Build history of the part. All positions in model axes, mm. A direction names the side the tool comes from. Round coordinates to 2 decimals unless told otherwise and drop trailing zeros. Loops run counter-clockwise (first coordinate to the right, second up) from the corner with the lowest first, then second, coordinate; pieces in that order, holes last. Notation, with made-up numbers: M 10,2 L 56,2 A14 cw 56,14 Z; hole C 1.25,65.5 d5. An arc over 180 degrees is marked long. Use one line per item in the form item = value. Start each with the question number.
```python
from build123d import *

# Parameters (mm, degrees)
F0_W     = 220.925912261
F0_H     = 147.3058909178
F1_DEPTH = 22.8
F2_W     = 170.8267480135
F2_H     = 112.4693089873
F3_DEPTH = 8.8
F5_D     = 11


with BuildPart() as f1:
    # F0 (on Top) → F1 (new body)
    with BuildSketch(Plane.XY):
        Rectangle(F0_W, F0_H)
    extrude(amount=F1_DEPTH)

    # F2 (on face) → F3 (cut)
    with BuildSketch(Plane.XY.offset(22.8)):
        Rectangle(F2_W, F2_H)
    extrude(amount=-F3_DEPTH, mode=Mode.SUBTRACT)

    # F5 (through all)
    with Locations(Plane.XY.offset(22.8)):
        with Locations((97.8735089302, 0)):
            Hole(F5_D / 2)


solid = f1.part
```
Q1. Tool access for faces 1 (the face through (-1, 56.235, 18)), 2 (the face through (-2, 73.653, 11)): list every direction of +Z, -Z, +X, -X, +Y, -Y with a clear straight run to the whole face (end or side of a thin tool).
Q2. Drop a flat-ended pin along its axis: P1, Ø3, axis at x = 21.5, y = 5, coming from the +Z side. Give the stop position or say it passes through.
Q3. Pull direction Y, two halves, no side cores. Call faces 3 (the face through (110.463, -1, 11)), 4 (the face through (-2, -73.653, 11)), 5 (the face through (-1, -56.235, 18)): pulls with the +Y half, pulls with the -Y half, needs draft (parallel to the pull), parting line crosses it, or undercut.
Q4. Saw through at B-B (x = -2.5). Give the cut face in (y, z), and give its area (3 significant figures).
Q5. Saw through at A-A (y = 16). Give the cut face in (x, z).
Q6. Wall check: probe 1 along X at (y, z) = (14.5, 21.5); probe 2 along Y at (x, z) = (-1, 18.5); probe 3 along Z at (x, y) = (11, 28). Give the ranges that are in metal, low to high.
Q7. Saw through at C-C (y = 0). Give the cut face in (x, z).
Filled in:
q1.face_1 = +Z
q1.face_2 = +Z, -Z, +X, -X, +Y
q2.P1 = 14
q3.face_3 = needs draft
q3.face_4 = pulls with the -Y half
q3.face_5 = undercut
q4.outline = M -73.65,0 L 73.65,0 L 73.65,22.8 L 56.23,22.8 L 56.23,14 L -56.23,14 L -56.23,22.8 L -73.65,22.8 Z
q4.area = 2,370 mm²
q5.outline = M -110.46,0 L 110.46,0 L 110.46,22.8 L 85.41,22.8 L 85.41,14 L -85.41,14 L -85.41,22.8 L -110.46,22.8 Z
q6.probe_1 = -110.46 to -85.41, 85.41 to 110.46
q6.probe_2 = -73.65 to -56.23, 56.23 to 73.65
q6.probe_3 = 0 to 14
q7.outline = M -110.46,0 L 92.37,0 L 92.37,22.8 L 85.41,22.8 L 85.41,14 L -85.41,14 L -85.41,22.8 L -110.46,22.8 Z; M 103.37,0 L 110.46,0 L 110.46,22.8 L 103.37,22.8 Z
